from build123d import *

# Parameters (mm, degrees)
ESQUISSE1_R             = 21.5
ESQUISSE1_R_2           = 1.7
ESQUISSE1_R_3           = 13.5
BOSS_EXTRU_1_DEPTH      = 8
BOSS_EXTRU_2_START      = -8
ESQUISSE2_R             = 5
BOSS_EXTRU_2_DEPTH      = 8
ENL_V_MAT_EXTRU_1_DEPTH = 111.605108381
CONG_1_R                = 6
ESQUISSE4_R             = 1.5
BOSS_EXTRU_3_DEPTH      = 8
ESQUISSE5_R             = 2.9
ENL_V_MAT_EXTRU_2_DEPTH = 3


with BuildPart() as part:
    # Esquisse1 → Boss.-Extru.1 (new body)
    with BuildSketch(Plane.XY):
        Circle(ESQUISSE1_R)
        with Locations((0, 17.5)):
            Circle(ESQUISSE1_R_2, mode=Mode.SUBTRACT)
        with Locations((17.5, 0)):
            Circle(ESQUISSE1_R_2, mode=Mode.SUBTRACT)
        with Locations((0, -17.5)):
            Circle(ESQUISSE1_R_2, mode=Mode.SUBTRACT)
        with Locations((-17.5, 0)):
            Circle(ESQUISSE1_R_2, mode=Mode.SUBTRACT)
        Circle(ESQUISSE1_R_3, mode=Mode.SUBTRACT)
    extrude(amount=BOSS_EXTRU_1_DEPTH)

    # Esquisse2 → Boss.-Extru.2 (add)
    with BuildSketch(Plane.XY.offset(8).offset(BOSS_EXTRU_2_START)):
        with BuildLine():
            Line((2.8595, 21.308994809), (101.0906, 8.127151508))
            ThreePointArc((101.0906, 8.127151508), (108.2, 0), (101.0906, -8.127151508))
            Line((101.0906, -8.127151508), (2.8595, -21.308994809))
            ThreePointArc((2.8595, -21.308994809), (21.5, 0), (2.8595, 21.308994809))
        make_face()
        with Locations((100, 0)):
            Circle(ESQUISSE2_R, mode=Mode.SUBTRACT)
    extrude(amount=BOSS_EXTRU_2_DEPTH)

    # Esquisse3 → Enlèv. mat.-Extru.1 (cut, through all)
    with BuildSketch(Plane.XY.offset(8)):
        with BuildLine():
            Line((14.706535342, 15.683361191), (93.578440575, 5.099370015))
            ThreePointArc((93.578440575, 5.099370015), (91.8, 0), (93.578440575, -5.099370015))
            Line((93.578440575, -5.099370015), (14.706535342, -15.683361191))
            ThreePointArc((14.706535342, -15.683361191), (21.5, 0), (14.706535342, 15.683361191))
        make_face()
    extrude(amount=-ENL_V_MAT_EXTRU_1_DEPTH, mode=Mode.SUBTRACT)

    # Congé1
    cong_1_edges = [part.edges().sort_by_distance(p)[0] for p in [
        (14.706535342, -15.683361191, 4),
        (14.706535342, 15.683361191, 4),
        (93.578440575, 5.099370015, 4),
        (93.578440575, -5.099370015, 4),
    ]]
    fillet(cong_1_edges, radius=CONG_1_R)

    # Esquisse4 → Boss.-Extru.3 (add)
    with BuildSketch(Plane.XY.offset(8)):
        with BuildLine():
            Line((103.69, 7.322834151), (116.45, 0.893028555))
            ThreePointArc((116.45, 0.893028555), (117, 0), (116.45, -0.893028555))
            Line((116.45, -0.893028555), (103.69, -7.322834151))
            ThreePointArc((103.69, -7.322834151), (108.2, 0), (103.69, 7.322834151))
        make_face()
        with Locations((110, 0)):
            Circle(ESQUISSE4_R, mode=Mode.SUBTRACT)
    extrude(amount=-BOSS_EXTRU_3_DEPTH)

    # Esquisse5 → Enlèv. mat.-Extru.2 (cut)
    with BuildSketch(Plane.XY.offset(8)):
        with Locations((0, 17.5)):
            Circle(ESQUISSE5_R)
        with Locations((17.5, 0)):
            Circle(ESQUISSE5_R)
        with Locations((0, -17.5)):
            Circle(ESQUISSE5_R)
        with Locations((-17.5, 0)):
            Circle(ESQUISSE5_R)
    extrude(amount=-ENL_V_MAT_EXTRU_2_DEPTH, mode=Mode.SUBTRACT)


solid = part.part
CAD build for the part. Positions are in the model's coordinates, mm. A direction names the side the tool comes from. Round coordinates to 2 decimals unless told otherwise and drop trailing zeros. Write each loop counter-clockwise with the first axis right and the second up, starting at its lowest first coordinate (ties: lowest second). Pieces come first, ordered by that corner, then holes. Notation, with made-up numbers: (69.5, 60) -> (85.5, 60) arc R13 cw to (85.5, 73) -> close; hole circle Ø4 at (23, -35). An arc over 180 degrees is marked (long way). Answer as a JSON object with one key per item and string values.
(1) Band-saw the part on D-D, the plane x = 17. List the corners of the cut face in (y, z), then the cut area to 3 significant figures.
Reported:
{"outline": "(-19.41, 0) -> (-1.62, 0) -> (-1.62, 5) -> (-2.86, 5) -> (-2.86, 8) -> (-19.41, 8) -> close; (1.62, 0) -> (19.41, 0) -> (19.41, 8) -> (2.86, 8) -> (2.86, 5) -> (1.62, 5) -> close", "area": "277 mm^2"}
(2) Probe probe 1 along Y at (x, z) = (0, 6.75); probe 2 along Y at (x, z) = (0, 3); probe 3 along X at (y, z) = (4, 5). List the from-to ranges inside material, lowest first. Write a range as [from, to].
Reported:
{"probe 1": "y = [-21.5, -20.4], [-14.6, -13.5], [13.5, 14.6], [20.4, 21.5]", "probe 2": "y = [-21.5, -19.2], [-15.8, -13.5], [13.5, 15.8], [19.2, 21.5]", "probe 3": "x = [-21.12, -12.89], [12.89, 21.12], [90.35, 97], [103, 110.28]"}
(3) Band-saw the part on B-B, the plane z = 2.5. Count the separate pieces of the cut face and the enclosed holes in it, then the cut area to 3 significant figures.
Reported:
{"separate pieces": "1", "enclosed holes": "8", "area": "1,790 mm^2"}
(4) Band-saw the part on A-A, the plane x = 0. List the corners of the cut face in (y, z), then the cut area to 3 significant figures.
Reported:
{"outline": "(-21.5, 0) -> (-19.2, 0) -> (-19.2, 5) -> (-20.4, 5) -> (-20.4, 8) -> (-21.5, 8) -> close; (-15.8, 0) -> (-13.5, 0) -> (-13.5, 8) -> (-14.6, 8) -> (-14.6, 5) -> (-15.8, 5) -> close; (13.5, 0) -> (15.8, 0) -> (15.8, 5) -> (14.6, 5) -> (14.6, 8) -> (13.5, 8) -> close; (19.2, 0) -> (21.5, 0) -> (21.5, 8) -> (20.4, 8) -> (20.4, 5) -> (19.2, 5) -> close", "area": "59.2 mm^2"}
(5) Which spindle directions (+Z, -Z, +X, -X, +Y, -Y) get a long thin tool onto all of the face, cutting with end or side? Do faces 1 (the face through (110.159, -4.063, 4.056)), 2 (the face through (-18, -2, 5)), 3 (the face through (90.37, 3.98, 3.94)). Say none if no direction does.
Reported:
{"face 1": "+Z, -Z, +X, -Y", "face 2": "+Z", "face 3": "+Z, -Z"}
(6) Pin check, flat tips, straight feed: P1, Ø1, axis at y = 6, z = 6.5, coming from the +X side; P2, Ø2, axis at x = -17.5, y = 0, coming from the +Z side; P3, Ø2, axis at x = 65.5, z = 2.5, coming from the +Y side; P4, Ø2, axis at y = -2, z = 1.5, coming from the +X side. Stop position of each tip, or through.
Reported:
{"P1": "stops at x = 107.31", "P2": "passes through", "P3": "stops at y = 13.04", "P4": "stops at x = 116.24"}
(7) Two-plate mould, pull along X, no slides. Class faces 4 (the face through (109.981, 4.153, 4.056)), 5 (the face through (14.6, 0.1, 6.5)), 6 (the face through (38, -13, 8)): +X half, -X half, draft (parallel to the pull), parting line (faces both ways), or undercut.
Reported:
{"face 4": "+X half", "face 5": "undercut", "face 6": "draft"}
(8) Band-saw the part on C-C, the plane y = -17.5. List the corners of the cut face in (x, z), then the cut area to 3 significant figures.
Reported:
{"outline": "(-12.49, 0) -> (-1.7, 0) -> (-1.7, 5) -> (-2.9, 5) -> (-2.9, 8) -> (-12.49, 8) -> close; (1.7, 0) -> (31.24, 0) -> (31.24, 8) -> (2.9, 8) -> (2.9, 5) -> (1.7, 5) -> close", "area": "315 mm^2"}
